The model under review builds one solid part; all positions refer to its coordinate system, in mm. Coordinates: 2 decimals unless noted, no trailing zeros. Loops run counter-clockwise (first coordinate to the right, second up) from the corner with the lowest first, then second, coordinate; pieces in that order, holes last. Notation, with made-up numbers: (0.5, 24) - (43.5, 24) arc R19 cw to (43.5, 35) - close; hole circle Ø9 at (-34, -25). An arc over 180 degrees is marked (long way). Answer in a Markdown table with one row per item. Add a question column.
(1) We need section C-C on z = 48. Write out the cut boundary in (x, y), plus the area to 3 significant figures.
(2) For P1, Ø0.9, axis at y = 2, z = -52, coming from the +X side, flat-tipped, find the tip position at first contact; note if it passes through.
(3) We need section D-D on y = 0.5. Give the number of separate pieces and of enclosed holes in the cut face, plus the area to 3 significant figures.
(4) We need section A-A on x = 55. Write out the cut boundary in (y, z).
(5) We need section B-B on z = -55. Write out the cut boundary in (x, y), plus the area to 3 significant figures.
(6) For line 1 along X through (y, z) = (1.5, -55); line 2 along X through (y, z) = (2.1, 55); line 3 along Z through (x, y) = (-28.5, 1.5), list the stretches that pass through material, from the lowest coordinate up.
from build123d import *

# Parameters (mm, degrees)
SZKIC1_R                    = 4
DODANIE_WYCI_GNI_CIE1_DEPTH = 3
ZAOKR_GLENIE1_R             = 10


with BuildPart() as part:
    # Szkic1 → Dodanie-wyciągnięcie1 (new body)
    with BuildSketch(Plane(origin=(0, 0, 0), x_dir=(1, 0, 0), z_dir=(0, 1, 0))):
        Polygon((77.5, -77.5), (120.801270189, -102.5), (170.801270189, -15.897459622), (77.5, 37.970053838), (77.5, 77.5), (-77.5, 77.5), (-77.5, -77.5), align=None)
        with Locations(Location((-55, 55, 0), (0, 0, 270))):
            Circle(SZKIC1_R, mode=Mode.SUBTRACT)
        with Locations(Location((55, 55, 0), (0, 0, 270))):
            Circle(SZKIC1_R, mode=Mode.SUBTRACT)
        with Locations(Location((55, -55, 0), (0, 0, 270))):
            Circle(SZKIC1_R, mode=Mode.SUBTRACT)
        with Locations(Location((-55, -55, 0), (0, 0, 270))):
            Circle(SZKIC1_R, mode=Mode.SUBTRACT)
        with Locations(Location((159.739092363, -21.057713659, 0), (0, 0, 270))):
            Circle(SZKIC1_R, mode=Mode.SUBTRACT)
        with Locations(Location((143.739092363, -48.770526581, 0), (0, 0, 270))):
            Circle(SZKIC1_R, mode=Mode.SUBTRACT)
        with Locations(Location((128.562177826, -3.057713659, 0), (0, 0, 90))):
            Circle(SZKIC1_R, mode=Mode.SUBTRACT)
        with Locations(Location((112.562177826, -30.770526581, 0), (0, 0, 90))):
            Circle(SZKIC1_R, mode=Mode.SUBTRACT)
    extrude(amount=DODANIE_WYCI_GNI_CIE1_DEPTH)

    # Zaokrąglenie1
    zaokr_glenie1_edges = [part.edges().sort_by_distance(p)[0] for p in [
        (-77.5, 1.5, -77.5),
        (77.5, 1.5, -77.5),
        (170.801270189, 1.5, 15.897459622),
        (120.801270189, 1.5, 102.5),
        (-77.5, 1.5, 77.5),
    ]]
    fillet(zaokr_glenie1_edges, radius=ZAOKR_GLENIE1_R)


solid = part.part
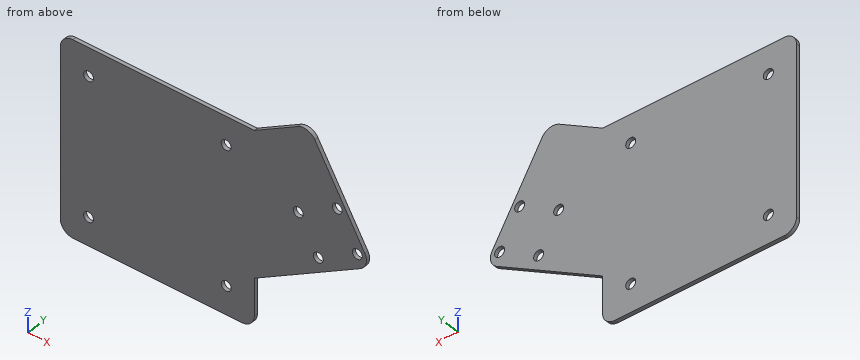
Outcome:
| question | item | result |
|---|---|---|
| 1 | outline | (-77.5, 0) - (139.81, 0) - (139.81, 3) - (-77.5, 3) - close; (147.66, 0) - (152.27, 0) - (152.27, 3) - (147.66, 3) - close |
| 1 | area | 666 mm² |
| 2 | P1 | x = 77.5 |
| 3 | separate pieces | 1 |
| 3 | enclosed holes | 8 |
| 3 | area | 31,400 mm² |
| 4 | outline | (0, -77.5) - (3, -77.5) - (3, -59) - (0, -59) - close; (0, -51) - (3, -51) - (3, 51) - (0, 51) - close; (0, 59) - (3, 59) - (3, 77.5) - (0, 77.5) - close |
| 5 | outline | (-77.5, 0) - (-59, 0) - (-59, 3) - (-77.5, 3) - close; (-51, 0) - (51, 0) - (51, 3) - (-51, 3) - close; (59, 0) - (77.5, 0) - (77.5, 3) - (59, 3) - close |
| 5 | area | 417 mm² |
| 6 | line 1 | -77.5 to -59, -51 to 51, 59 to 77.5 |
| 6 | line 2 | -77.5 to -59, -51 to 51, 59 to 148.23 |
| 6 | line 3 | -77.5 to 77.5 |
